Here's how the part is built. I have some questions about the finished solid (model axes, mm). Face numbers are marked on the shaded views. A direction names the side the tool comes from. Round coordinates to 2 decimals unless told otherwise and drop trailing zeros. Loops run counter-clockwise (first coordinate to the right, second up) from the corner with the lowest first, then second, coordinate; pieces in that order, holes last. Notation, with made-up numbers: (39, 33) -> (55, 33) arc R20 ccw to (55, 65) -> close; hole circle Ø11 at (-26, 36.5). An arc over 180 degrees is marked (long way). Use one line per item in the form item = value. Start each with the question number.
Item 1: Thinking about a two-plate mould opening in Y: for the marked faces 4, 5 and 6, which applies, released by +Y, released by -Y, zero draft, split by the parting line, or undercut?
Item 2: For the marked faces 1, 2 and 3, which set-ups out of +Z, -Z, +X, -X, +Y, -Y let a thin tool reach every point of the face, with its end or its side?
Item 3: I'm going to push a flat-ended pin straight in: pin 1 Ø9.5 at (x, y) = (-60, 1) entering from +Z. Where does the tip first touch, or does it pass through?
Item 4: If we section it at D-D (y = 8.5): Write out the boundary of the cut face in (x, z), then the cut area to 3 significant figures.
Item 5: If I drill on L1, parallel to Y at x = -58.5, z = 3.25; L2, parallel to X at y = -10, z = 7.75; L3, parallel to Y at x = -71, z = 4.5, over which ranges is the centre line in solid material (lowest first)? Write a range as [from, to].
Item 6: If we section it at A-A (y = -10.75): Write out the boundary of the cut face in (x, z).
Item 7: If we section it at B-B (x = -54.5): Write out the boundary of the cut face in (y, z), then the cut area to 3 significant figures.
Item 8: If we section it at C-C (z = 4): Write out the boundary of the cut face in (x, y), then the cut area to 3 significant figures.
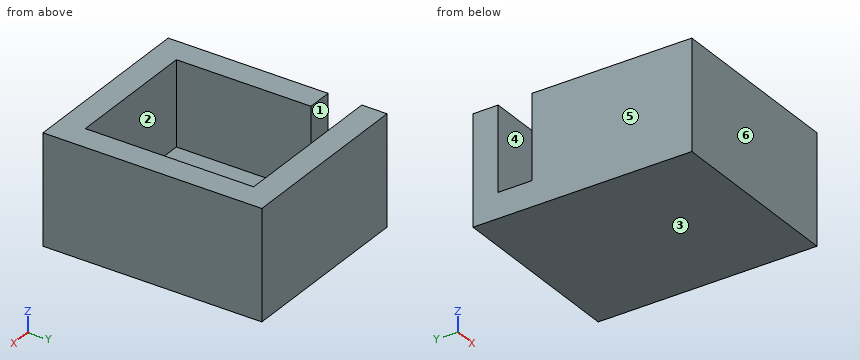
```python
from build123d import *

# Parameters (mm, degrees)
BOSS_EXTRUDE1_DEPTH = 10
SKETCH2_W           = 22
SKETCH2_H           = 26
BOSS_EXTRUDE2_DEPTH = 3


with BuildPart() as part:
    # Sketch1 → Boss-Extrude1 (new body)
    with BuildSketch(Plane.XY):
        Polygon((-72.1, 8.9), (-53.1, 8.9), (-53.1, -11.1), (-69.1, -11.1), (-69.1, 4.9), (-72.1, 4.9), (-72.1, -14.1), (-50.1, -14.1), (-50.1, 11.9), (-72.1, 11.9), align=None)
    extrude(amount=BOSS_EXTRUDE1_DEPTH)

    # Sketch2 → Boss-Extrude2 (add)
    with BuildSketch(Plane(origin=(0, 0, 0), x_dir=(-1, 0, 0), z_dir=(0, 0, -1))):
        with Locations((61.1, -1.1)):
            Rectangle(SKETCH2_W, SKETCH2_H)
    extrude(amount=BOSS_EXTRUDE2_DEPTH)


solid = part.part
```
Values found:
q1.face_4 = undercut
q1.face_5 = zero draft
q1.face_6 = released by -Y
q2.face_1 = +Z, -X
q2.face_2 = +Z
q2.face_3 = -Z, +X, -X, +Y, -Y
q3.pin_1 = 0
q4.outline = (-72.1, -3) -> (-50.1, -3) -> (-50.1, 10) -> (-53.1, 10) -> (-53.1, 0) -> (-72.1, 0) -> close
q4.area = 96.0 mm2
q5.L1 = [-14.1, -11.1], [8.9, 11.9]
q5.L2 = [-72.1, -69.1], [-53.1, -50.1]
q5.L3 = [-14.1, 4.9], [8.9, 11.9]
q6.outline = (-72.1, -3) -> (-50.1, -3) -> (-50.1, 10) -> (-53.1, 10) -> (-53.1, 0) -> (-69.1, 0) -> (-69.1, 10) -> (-72.1, 10) -> close
q7.outline = (-14.1, -3) -> (11.9, -3) -> (11.9, 10) -> (8.9, 10) -> (8.9, 0) -> (-11.1, 0) -> (-11.1, 10) -> (-14.1, 10) -> close
q7.area = 138 mm2
q8.outline = (-72.1, -14.1) -> (-50.1, -14.1) -> (-50.1, 11.9) -> (-72.1, 11.9) -> (-72.1, 8.9) -> (-53.1, 8.9) -> (-53.1, -11.1) -> (-69.1, -11.1) -> (-69.1, 4.9) -> (-72.1, 4.9) -> close
q8.area = 240 mm2
